Source: CAD feature listing. Evaluate the final solid. Frame: model axes, mm. A direction names the side the tool comes from. Coordinates: 2 decimals unless noted, no trailing zeros. Order: outer loops, then holes, each group sorted by start corner. A loop starts at its lowest first (then second) coordinate and runs counter-clockwise, first axis right, second up.
```python
from build123d import *

# Parameters (mm, degrees)
SKETCH_1_W          = 100
SKETCH_1_H          = 50
SKETCH_1_W_2        = 95
SKETCH_1_H_2        = 46
EXTRUDE_1_DEPTH     = 19.5
SKETCH_2_R          = 1.6
CUT_EXTRUDE_1_DEPTH = 51
CUT_EXTRUDE_2_REACH = 102
SKETCH_3_R          = 10.25
SKETCH_3_R_2        = 2.15
SKETCH_3_R_3        = 1.6
CUT_EXTRUDE_3_REACH = 102
SKETCH_4_R          = 12.5


with BuildPart() as part:
    # ｽｹｯﾁ1 → ﾎﾞｽ - 押し出し1 (new body, symmetric)
    with BuildSketch(Plane.XY):
        Rectangle(SKETCH_1_W, SKETCH_1_H)
        Rectangle(SKETCH_1_W_2, SKETCH_1_H_2, mode=Mode.SUBTRACT)
    extrude(amount=EXTRUDE_1_DEPTH, both=True)

    # ｽｹｯﾁ2 → ｶｯﾄ - 押し出し1 (cut, through all)
    with BuildSketch(Plane(origin=(0, 25, 0), x_dir=(1, 0, 0), z_dir=(0, 1, 0))):
        with Locations((-15, 15.820888862)):
            Circle(SKETCH_2_R)
        with Locations((10.711504387, -14.820888862)):
            Circle(SKETCH_2_R)
    extrude(amount=-CUT_EXTRUDE_1_DEPTH, mode=Mode.SUBTRACT)

    # ｽｹｯﾁ3 → ｶｯﾄ - 押し出し2 (cut, up to next)
    with BuildSketch(Plane.ZY.offset(50), mode=Mode.PRIVATE) as cut_extrude_2_sk1:
        with Locations((4.5, 0)):
            Circle(SKETCH_3_R)
    cut_extrude_2_tool1 = extrude(cut_extrude_2_sk1.sketch, amount=-CUT_EXTRUDE_2_REACH, mode=Mode.PRIVATE) & part.part
    add(cut_extrude_2_tool1.solids().sort_by_distance((-50, 0, 4.5))[0], mode=Mode.SUBTRACT)
    # ｽｹｯﾁ3 → ｶｯﾄ - 押し出し2 (cut, up to next)
    with BuildSketch(Plane.ZY.offset(50), mode=Mode.PRIVATE) as cut_extrude_2_sk2:
        with Locations((-12.5, 0)):
            Circle(SKETCH_3_R_2)
    cut_extrude_2_tool2 = extrude(cut_extrude_2_sk2.sketch, amount=-CUT_EXTRUDE_2_REACH, mode=Mode.PRIVATE) & part.part
    add(cut_extrude_2_tool2.solids().sort_by_distance((-50, 0, -12.5))[0], mode=Mode.SUBTRACT)
    # ｽｹｯﾁ3 → ｶｯﾄ - 押し出し2 (cut, up to next)
    with BuildSketch(Plane.ZY.offset(50), mode=Mode.PRIVATE) as cut_extrude_2_sk3:
        with Locations((13, 14.722431864)):
            Circle(SKETCH_3_R_2)
    cut_extrude_2_tool3 = extrude(cut_extrude_2_sk3.sketch, amount=-CUT_EXTRUDE_2_REACH, mode=Mode.PRIVATE) & part.part
    add(cut_extrude_2_tool3.solids().sort_by_distance((-50, 14.722432, 13))[0], mode=Mode.SUBTRACT)
    # ｽｹｯﾁ3 → ｶｯﾄ - 押し出し2 (cut, up to next)
    with BuildSketch(Plane.ZY.offset(50), mode=Mode.PRIVATE) as cut_extrude_2_sk4:
        with Locations((13, -14.722431864)):
            Circle(SKETCH_3_R_2)
    cut_extrude_2_tool4 = extrude(cut_extrude_2_sk4.sketch, amount=-CUT_EXTRUDE_2_REACH, mode=Mode.PRIVATE) & part.part
    add(cut_extrude_2_tool4.solids().sort_by_distance((-50, -14.722432, 13))[0], mode=Mode.SUBTRACT)
    # ｽｹｯﾁ3 → ｶｯﾄ - 押し出し2 (cut, up to next)
    with BuildSketch(Plane.ZY.offset(50), mode=Mode.PRIVATE) as cut_extrude_2_sk5:
        with Locations((-14.5, -17)):
            Circle(SKETCH_3_R_3)
    cut_extrude_2_tool5 = extrude(cut_extrude_2_sk5.sketch, amount=-CUT_EXTRUDE_2_REACH, mode=Mode.PRIVATE) & part.part
    add(cut_extrude_2_tool5.solids().sort_by_distance((-50, -17, -14.5))[0], mode=Mode.SUBTRACT)
    # ｽｹｯﾁ3 → ｶｯﾄ - 押し出し2 (cut, up to next)
    with BuildSketch(Plane.ZY.offset(50), mode=Mode.PRIVATE) as cut_extrude_2_sk6:
        with Locations((-14.5, 17)):
            Circle(SKETCH_3_R_3)
    cut_extrude_2_tool6 = extrude(cut_extrude_2_sk6.sketch, amount=-CUT_EXTRUDE_2_REACH, mode=Mode.PRIVATE) & part.part
    add(cut_extrude_2_tool6.solids().sort_by_distance((-50, 17, -14.5))[0], mode=Mode.SUBTRACT)

    # ｽｹｯﾁ4 → ｶｯﾄ - 押し出し3 (cut, up to next)
    with BuildSketch(Plane(origin=(50, 0, 0), x_dir=(0, 0, -1), z_dir=(1, 0, 0)), mode=Mode.PRIVATE) as cut_extrude_3_sk1:
        with Locations((-4.5, 0)):
            Circle(SKETCH_4_R)
    cut_extrude_3_tool1 = extrude(cut_extrude_3_sk1.sketch, amount=-CUT_EXTRUDE_3_REACH, mode=Mode.PRIVATE) & part.part
    add(cut_extrude_3_tool1.solids().sort_by_distance((50, 0, 4.5))[0], mode=Mode.SUBTRACT)


solid = part.part
```
Q1. Set-up query: faces 4 (the flat face through (-1, 23, 0)), 5 (the cylindrical face through (48.768, 3.755, -7.423)), 6 (the cylindrical face through (-48.77, -15.92, -15.68)), 7 (the flat face through (-1, -25, 0)), 8 (the cylindrical face through (-16.27, -23.99, -14.85)). Return all of +Z, -Z, +X, -X, +Y, -Y with unobstructed straight access to the full face (end or side cutting, diameter ignored); none if empty.
Solutions:
face 4: +Z, -Z
face 5: +X
face 6: -X
face 7: +Z, -Z, +X, -X, -Y
face 8: +Y, -Y
Q2. Pin query (flat end, axial travel): P1, Ø3.5, axis at y = 14.72, z = 13, coming from the -X side; P2, Ø4, axis at y = -8.5, z = 9, coming from the +X side. Return the tip coordinate at first contact, or that it passes through.
Solutions:
P1: stops at x = 47.5
P2: stops at x = -47.5
Q3. Material intervals for line 1 along X through (y, z) = (19.5, -8); line 2 along Y through (x, z) = (-13, 4.5); line 3 along Y through (x, z) = (-48, 13), sorted ascending.
Solutions:
line 1: x = -50 to -47.5, 47.5 to 50
line 2: y = -25 to -23, 23 to 25
line 3: y = -25 to -16.87, -12.57 to -5.73, 5.73 to 12.57, 16.87 to 25
Q4. Section query B-B on y = 21. Output: boundary loops of the cut face in (x, z), plus the area to 3 significant figures.
Solutions:
outline: (-50, -19.5) - (-47.5, -19.5) - (-47.5, 19.5) - (-50, 19.5) - close; (47.5, -19.5) - (50, -19.5) - (50, 19.5) - (47.5, 19.5) - close
area: 195 mm2
Q5. Section query D-D on z = 4.5. Output: boundary loops of the cut face in (x, y), plus the area to 3 significant figures.
Solutions:
outline: (-50, -25) - (50, -25) - (50, -12.5) - (47.5, -12.5) - (47.5, -23) - (-47.5, -23) - (-47.5, -10.25) - (-50, -10.25) - close; (-50, 10.25) - (-47.5, 10.25) - (-47.5, 23) - (47.5, 23) - (47.5, 12.5) - (50, 12.5) - (50, 25) - (-50, 25) - close
area: 516 mm2
Q6. Pull-direction query (Y, two-part tool) for faces 1 (the flat face through (-1, 25, 0)), 2 (the cylindrical face through (-16.27, 24.01, -14.85)), 3 (the cylindrical face through (-48.77, 18.08, -15.68)); classes: pulls with the +Y half, pulls with the -Y half, needs draft (parallel to the pull), parting line crosses it, or undercut.
Solutions:
face 1: pulls with the +Y half
face 2: needs draft
face 3: undercut
Q7. Section query A-A on x = -15. Output: boundary loops of the cut face in (y, z).
Solutions:
outline: (-25, -19.5) - (-23, -19.5) - (-23, -17.42) - (-25, -17.42) - close; (-25, -14.22) - (-23, -14.22) - (-23, 19.5) - (-25, 19.5) - close; (23, -19.5) - (25, -19.5) - (25, -17.42) - (23, -17.42) - close; (23, -14.22) - (25, -14.22) - (25, 19.5) - (23, 19.5) - close
Q8. Section query C-C on x = 42.5. Output: boundary loops of the cut face in (y, z), plus the area to 3 significant figures.
Solutions:
outline: (-25, -19.5) - (-23, -19.5) - (-23, 19.5) - (-25, 19.5) - close; (23, -19.5) - (25, -19.5) - (25, 19.5) - (23, 19.5) - close
area: 156 mm2
